The drawing under review shows one solid part. Ordinate dimensions are in mm from its lowest x, y, z. A direction names the side the tool comes from. Coordinates: 2 decimals unless noted, no trailing zeros. Loops run counter-clockwise (first coordinate to the right, second up) from the corner with the lowest first, then second, coordinate; pieces in that order, holes last. Notation, with made-up numbers: M -18.75,-39 L -6.75,-39 A31 ccw -6.75,-2 Z; hole C 9,62.5 d7. An arc over 180 degrees is marked long. Answer as a JSON object with one key per item and string values. Group by question number.
1. Machinability: for the marked faces 1, 2 and 3, which of the approach directions +Z, -Z, +X, -X, +Y, -Y give a long, thin tool a straight path to every point of the face, cutting with its end or side? Answer none if there is none.
2. Consider section D-D (z = 63.5). State the section outline as (x, y) points.
3. Consider section C-C (z = 32.5). State the section outline as (x, y) points, then the cut area to 3 significant figures.
4. To check wall thickness, follow probe 1 along Y at (x, z) = (1.75, 20); probe 2 along Z at (x, y) = (4.25, 7.5); probe 3 along X at (y, z) = (3.75, 28). State the ranges of each line that lie inside material, in increasing order.
5. Insertion check: pin 1 (1.5 mm diameter, centred on x = 5, y = 1, fed in from -Z); pin 2 (1 mm diameter, centred on x = 6.5, z = 44.5, fed in from -Y); pin 3 (1 mm diameter, centred on y = 1.5, z = 13, fed in from +X); pin 4 (1 mm diameter, centred on x = 5.5, z = 41, fed in from -Y). Each pin has a flat end and moves straight along its axis. Give the tip position at first contact, or say it passes through.
6. Consider section A-A (x = 4). State the section outline as (y, z) points.
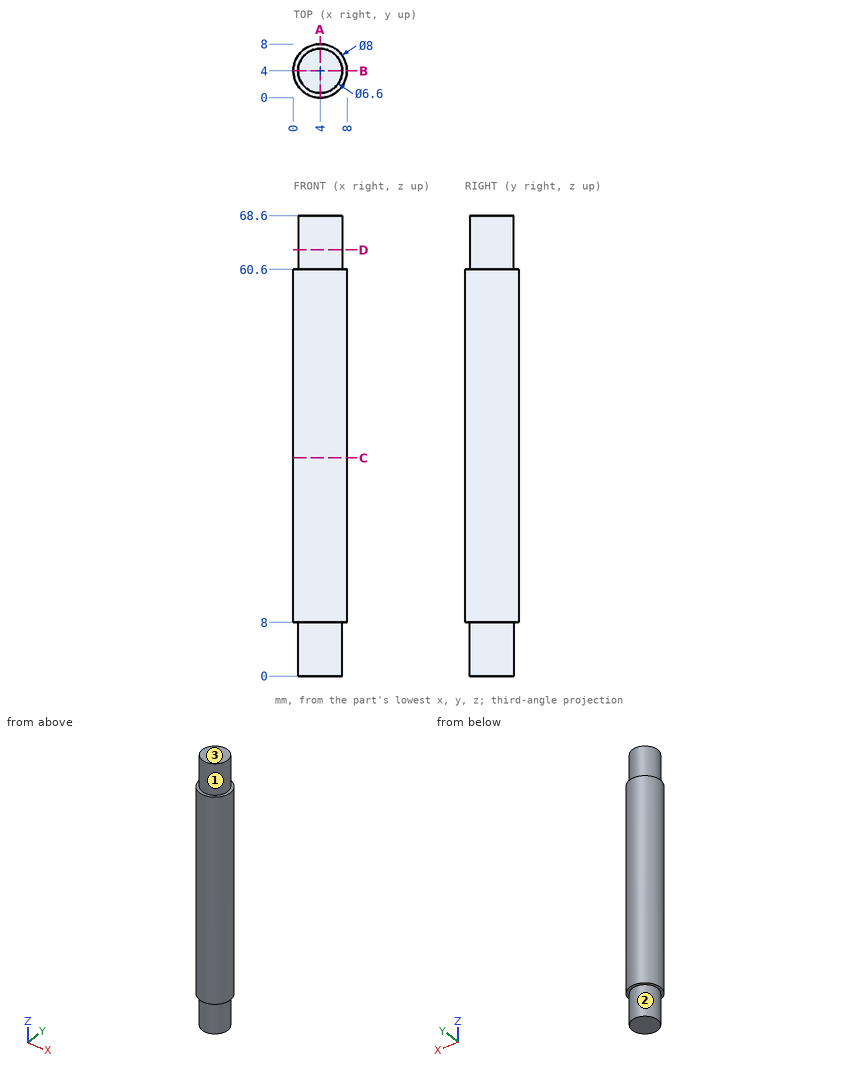
Findings below:
{
 "1": {"face 1": "+Z", "face 2": "-Z", "face 3": "+Z, +X, -X, +Y, -Y"},
 "2": {"outline": "C 4,4 d6.6"},
 "3": {"outline": "C 4,4 d8", "area": "50.3 mm^2"},
 "4": {"probe 1": "y = 0.69 to 7.31", "probe 2": "z = 8 to 60.6", "probe 3": "x = 0.01 to 7.99"},
 "5": {"pin 1": "stops at z = 0", "pin 2": "stops at y = 0.54", "pin 3": "stops at x = 7.46", "pin 4": "stops at y = 0.13"},
 "6": {"outline": "M 0,8 L 0.7,8 L 0.7,0 L 7.3,0 L 7.3,8 L 8,8 L 8,60.6 L 7.3,60.6 L 7.3,68.6 L 0.7,68.6 L 0.7,60.6 L 0,60.6 Z"}
}
